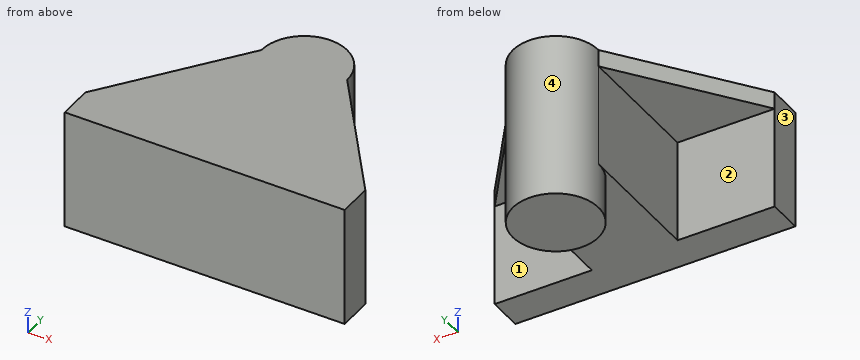
```python
from build123d import *

# Parameters (mm, degrees)
MAIN_BODY_DEPTH = 10.5
RIB1_REACH      = 45.385
SKETCH2_WALL_W  = 117.37050971
SKETCH2_WALL_H  = 3
SKETCH3_R       = 7.5
SHAFT_DEPTH     = 8


with BuildPart() as part:
    # Sketch1 → Main Body (new, symmetric)
    with BuildSketch(Plane.XY):
        with BuildLine():
            Line((-7.5, 0), (-7.5, -29))
            Line((-7.5, -29), (24.5, -29))
            Line((24.5, -29), (24.5, -23))
            Line((24.5, -23), (7.5, -23))
            Line((7.5, -23), (7.5, 0))
            ThreePointArc((7.5, 0), (0, 7.5), (-7.5, 0))
        make_face()
    main_body = extrude(amount=MAIN_BODY_DEPTH, both=True)

    # Sketch2 wall → Rib1 (add, up to next)
    with BuildSketch(Plane(origin=(16, -11.5, 10.5), x_dir=(0.594391061084, -0.804176141466, 0), z_dir=(0.804176141466, 0.594391061084, 0)), mode=Mode.PRIVATE) as rib1_sk1:
        with Locations((0, 1.5)):
            Rectangle(SKETCH2_WALL_W, SKETCH2_WALL_H)
    rib1_tool1 = extrude(rib1_sk1.sketch, amount=-RIB1_REACH, mode=Mode.PRIVATE) - part.part
    rib1 = rib1_tool1.solids().sort_by_distance((16, -11.5, 10.5))[0]
    add(rib1)

    # Sketch3 → Shaft (add)
    with BuildSketch(Plane.XY.offset(-10.5)):
        Circle(SKETCH3_R)
    extrude(amount=-SHAFT_DEPTH)

    # Mirror2: Main Body, Rib1 across plane
    add(main_body.mirror(Plane(origin=(0, 0, 0), x_dir=(0, 0, 1), z_dir=(1, 0, 0))))
    add(rib1.mirror(Plane(origin=(0, 0, 0), x_dir=(0, 0, 1), z_dir=(1, 0, 0))))


solid = part.part
```
Work out the finished part from the listing and answer in its coordinate system (mm). Face numbers are marked on the shaded views. A direction names the side the tool comes from. Round coordinates to 2 decimals unless told otherwise and drop trailing zeros. Write each loop counter-clockwise with the first axis right and the second up, starting at its lowest first coordinate (ties: lowest second). Pieces come first, ordered by that corner, then holes.
1) Which of the six approach directions +Z, -Z, +X, -X, +Y, -Y give full straight-line access (tool end or side, diameter ignored) to the marked faces 1, 2, 3 and 4?
2) A cutting plane is placed at D-D on x = -17.5. Determine the outline of the cut face in (y, z), and give its area (3 significant figures).
3) Flat-ended cylindrical pins translate along their axes: P1, Ø14.5, axis at y = -15.5, z = -1, coming from the +X side; P2, Ø6, axis at x = -19, y = -19.5, coming from the -Z side; P3, Ø14.5, axis at x = 11, y = -21.5, coming from the -Z side. Find the tip coordinate at first contact, or state that the pin passes through.
4) Consider probe 1 along Y at (x, z) = (-14, 3); probe 2 along X at (y, z) = (-6.5, 1.25); probe 3 along Z at (x, y) = (20, -24). Determine where each line is inside the solid, lowest interval first.
5) A cutting plane is placed at C-C on y = -8.5. Determine the outline of the cut face in (x, z).
6) A cutting plane is placed at B-B on z = -5.25. Determine the outline of the cut face in (x, y).
7) A cutting plane is placed at A-A on x = 0. Determine the outline of the cut face in (y, z), and give its area (4 significant figures).
Entries:
1. face 1: -Z, +X, +Y
1. face 2: -Z, -X, +Y
1. face 3: +Z, -Z, -X, +Y, -Y
1. face 4: -Z
2. outline: (-29, -10.5) - (-23, -10.5) - (-23, 7.5) - (-13.53, 7.5) - (-13.53, 10.5) - (-29, 10.5) - close
2. area: 154 mm2
3. P1: stops at x = 7.5
3. P2: stops at z = 7.5
3. P3: stops at z = -10.5
4. probe 1: y = -29 to -23
4. probe 2: x = -7.5 to 7.5
4. probe 3: z = -10.5 to 10.5
5. outline: (-13.78, 7.5) - (-7.5, 7.5) - (-7.5, -10.5) - (7.5, -10.5) - (7.5, 7.5) - (13.78, 7.5) - (13.78, 10.5) - (-13.78, 10.5) - close
6. outline: (-24.5, -29) - (24.5, -29) - (24.5, -23) - (7.5, -23) - (7.5, 0) arc R7.5 ccw to (-7.5, 0) - (-7.5, -23) - (-24.5, -23) - close
7. outline: (-29, -10.5) - (-7.5, -10.5) - (-7.5, -18.5) - (7.5, -18.5) - (7.5, 10.5) - (-29, 10.5) - close
7. area: 886.5 mm2
